Read the model definition and answer for the solid it produces. Units are mm, in the model's axes. A direction names the side the tool comes from. Coordinates: 2 decimals unless noted, no trailing zeros. Loops run counter-clockwise (first coordinate to the right, second up) from the corner with the lowest first, then second, coordinate; pieces in that order, holes last. Notation, with made-up numbers: (2, -38) -> (39, -38) arc R8 cw to (39, -25) -> close; hole circle Ø3 at (17, -11.75). An arc over 180 degrees is marked (long way). Answer as a JSON object with one key per item and string values. Group by question number.
1) Section B-B, the plane z = 4 is taken. Give the vertices of the cut face in (x, y).
2) Determine the mould class of faces 5 (the face through (1.972, -9.448, 21.537)), 6 (the face through (13, -5, 0)), 7 (the face through (-3, -12.8, 5)), 8 (the face through (-2.92, -6.99, 11.11)) for opening direction Z: released by +Z, released by -Z, zero draft, split by the parting line, or undercut.
3) Section D-D, the plane z = 20 is taken. Give the vertices of the cut face in (x, y), plus the area to 3 significant figures.
4) Consider probe 1 along Z at (x, y) = (45, -4.25); probe 2 along Y at (x, z) = (13.5, 6); probe 3 along X at (y, z) = (-4.5, 18). Determine where each line is inside the solid, lowest interval first. Write a range as [from, to].
5) Flat-ended cylindrical pins translate along their axes: P1, Ø6, axis at x = -2, z = 8.5, coming from the +Y side; P2, Ø4.5, axis at x = -2.5, z = 7, coming from the -Y side; P3, Ø2.5, axis at y = -9.65, z = 20, coming from the -X side; P4, Ø10, axis at x = 42.5, z = 18.5, coming from the -Y side. Find the tip coordinate at first contact, or state that the pin passes through.
6) Section A-A, the plane y = -9.65 is taken. Give the vertices of the cut face in (x, z).
7) Which of the six approach directions +Z, -Z, +X, -X, +Y, -Y give full straight-line access (tool end or side, diameter ignored) to faces 1 (the face through (-3, -6.5, 36)), 2 (the face through (31, -3.6, 16)), 3 (the face through (-3, -10, 32)), 4 (the face through (37, -5, 39))?
8) Section C-C, the plane x = 45 is taken. Give the vertices of the cut face in (y, z).
from build123d import *

# Parameters (mm, degrees)
SKETCH_W        = 50
SKETCH_H        = 40
PAD_DEPTH       = 15
SKETCH001_R     = 1.45
POCKET_DEPTH    = 12
POCKET001_DEPTH = 3.6
SKETCH003_W     = 6
SKETCH003_H     = 2
POCKET002_DEPTH = 15
SKETCH004_W     = 6.3
SKETCH004_H     = 8
PAD001_DEPTH    = 6.5
SKETCH005_W     = 70
SKETCH005_H     = 60
POCKET003_DEPTH = 9
SKETCH006_R     = 1.55
POCKET004_DEPTH = 5
SKETCH018_W     = 3
SKETCH018_H     = 3
POCKET010_DEPTH = 22
POCKET011_DEPTH = 6
PAD007_DEPTH    = 6.3
CHAMFER_SIZE    = 1


with BuildPart() as part:
    # Sketch (on XZ_Plane of Origin) → Pad (new body)
    with BuildSketch(Plane.XZ):
        with Locations((25, 20)):
            Rectangle(SKETCH_W, SKETCH_H)
    extrude(amount=PAD_DEPTH)

    # Sketch001 (on Face5 of Pad) → Pocket (cut)
    with BuildSketch(Plane(origin=(0, 0, 0), x_dir=(-1, 0, 0), z_dir=(0, 1, 0))):
        with Locations((-45, 4)):
            Circle(SKETCH001_R)
        with Locations((-15, 4)):
            Circle(SKETCH001_R)
    extrude(amount=-POCKET_DEPTH, mode=Mode.SUBTRACT)

    # Sketch002 (on Face4 of Pocket) → Pocket001 (cut)
    with BuildSketch(Plane(origin=(0, 0, 0), x_dir=(-1, 0, 0), z_dir=(0, 1, 0))):
        Polygon((-2.5, 0), (-56.5, 0), (-56.5, 40), (-27.253439, 40), (-2.5, 10.5), align=None)
    extrude(amount=-POCKET001_DEPTH, mode=Mode.SUBTRACT)

    # Sketch003 (on Face4 of Pocket001) → Pocket002 (cut)
    with BuildSketch(Plane(origin=(0, 0, 0), x_dir=(-1, 0, 0), z_dir=(0, 1, 0))):
        with Locations((-40, 39)):
            Rectangle(SKETCH003_W, SKETCH003_H)
    extrude(amount=-POCKET002_DEPTH, mode=Mode.SUBTRACT)

    # Sketch004 (on Face1 of Pocket002) → Pad001 (join)
    with BuildSketch(Plane(origin=(0, 0, 0), x_dir=(0, -1, 0), z_dir=(-1, 0, 0))):
        with Locations((9.65, 4)):
            Rectangle(SKETCH004_W, SKETCH004_H)
        with Locations((9.65, 36)):
            Rectangle(SKETCH004_W, SKETCH004_H)
    extrude(amount=PAD001_DEPTH)

    # Sketch005 (on Face6 of Pad001) → Pocket003 (cut)
    with BuildSketch(Plane.XZ.offset(15)):
        with Locations((39, 22)):
            Rectangle(SKETCH005_W, SKETCH005_H)
    extrude(amount=-POCKET003_DEPTH, mode=Mode.SUBTRACT)

    # Sketch006 (on Face1 of Pocket003) → Pocket004 (cut)
    with BuildSketch(Plane(origin=(0, 0, 0), x_dir=(0, -1, 0), z_dir=(-1, 0, 0))):
        with Locations((9.65, 20)):
            Circle(SKETCH006_R)
    extrude(amount=-POCKET004_DEPTH, mode=Mode.SUBTRACT)

    # Sketch018 (on Face21 of Pocket004) → Pocket010 (cut)
    with BuildSketch(Plane.YZ.offset(50)):
        with Locations((-0.3, 38.5)):
            Rectangle(SKETCH018_W, SKETCH018_H)
    extrude(amount=-POCKET010_DEPTH, mode=Mode.SUBTRACT)

    # Sketch019 (on Face15 of Pocket010) → Pocket011 (cut)
    with BuildSketch(Plane.YZ.offset(37)):
        Polygon((-6, 38), (-3.6, 36.5), (-3.6, 38), align=None)
    extrude(amount=POCKET011_DEPTH, mode=Mode.SUBTRACT)

    # Sketch020 (on Face10 of Pocket011) → Pad007 (join)
    with BuildSketch(Plane.XZ.offset(12.8)):
        Polygon((0, 8), (-6.5, 8), (0, 15), align=None)
    extrude(amount=-PAD007_DEPTH)

    # Chamfer
    chamfer_edges = [part.edges().sort_by_distance(p)[0] for p in [
        (-6.5, -12.8, 4),
        (-6.5, -6.5, 4),
        (-6.5, -12.8, 36),
        (-6.5, -6.5, 36),
        (-3.25, -12.8, 11.5),
        (-3.25, -6.5, 11.5),
    ]]
    chamfer(chamfer_edges, length=CHAMFER_SIZE)


solid = part.part
Determined:
{
 "1": {"outline": "(-6.5, -11.8) -> (-5.5, -12.8) -> (0, -12.8) -> (0, -15) -> (4, -15) -> (4, -6) -> (13.55, -6) -> (13.55, -3.6) -> (2.5, -3.6) -> (2.5, 0) -> (0, 0) -> (0, -6.5) -> (-5.5, -6.5) -> (-6.5, -7.5) -> close; (16.45, -6) -> (43.55, -6) -> (43.55, -3.6) -> (16.45, -3.6) -> close; (46.45, -6) -> (50, -6) -> (50, -3.6) -> (46.45, -3.6) -> close"},
 "2": {"face 5": "undercut", "face 6": "released by -Z", "face 7": "zero draft", "face 8": "undercut"},
 "3": {"outline": "(0, -15) -> (4, -15) -> (4, -11.2) -> (0, -11.2) -> close; (0, -8.1) -> (4, -8.1) -> (4, -6) -> (50, -6) -> (50, -3.6) -> (10.47, -3.6) -> (10.47, 0) -> (0, 0) -> close", "area": "181 mm²"},
 "4": {"probe 1": "[0, 2.55], [5.45, 40]", "probe 2": "[-6, -3.6]", "probe 3": "[0, 50]"},
 "5": {"P1": "y = 0", "P2": "y = -12.8", "P3": "through", "P4": "y = -6"},
 "6": {"outline": "(-6.5, 0) -> (4, 0) -> (4, 18.45) -> (0, 18.45) -> (0, 15) -> (-6.5, 8) -> close; (-6.5, 32) -> (0, 32) -> (0, 21.55) -> (4, 21.55) -> (4, 40) -> (-6.5, 40) -> close"},
 "7": {"face 1": "+Z, -Z, -X, +Y", "face 2": "-Z, +X, +Y", "face 3": "-X, +Y, -Y", "face 4": "+Z, +Y"},
 "8": {"outline": "(-6, 0) -> (-3.6, 0) -> (-3.6, 2.55) -> (-6, 2.55) -> close; (-6, 5.45) -> (-3.6, 5.45) -> (-3.6, 40) -> (-6, 40) -> close"}
}
